Can you work these out from the drawing? Everything is in mm from the part's minimum corner. A direction names the side the tool comes from. Coordinates: 2 decimals unless noted, no trailing zeros. Loops run counter-clockwise (first coordinate to the right, second up) from the corner with the lowest first, then second, coordinate; pieces in that order, holes last.
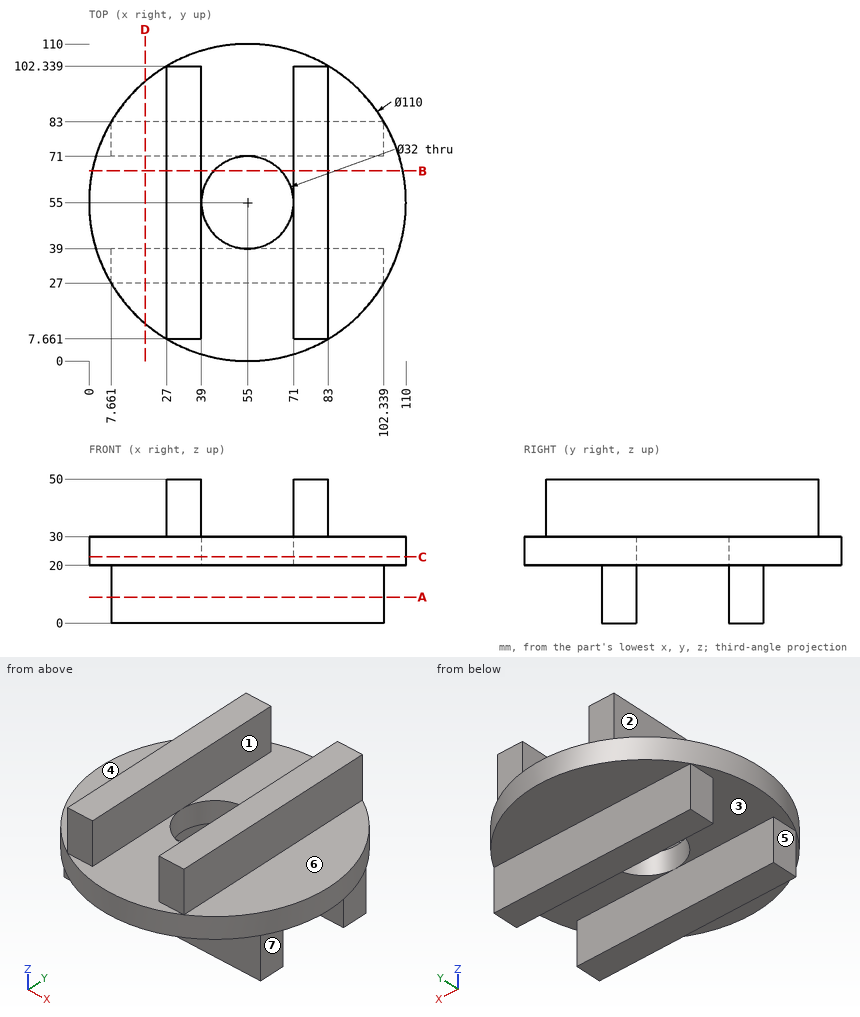
Item 1: Suppose I cut it at A-A, the plane z = 9. Please give me the cut outline in (x, y), plus the area to 3 significant figures.
Results are:
outline: (7.66, 27) - (102.34, 27) - (102.34, 39) - (7.66, 39) - close; (7.66, 71) - (102.34, 71) - (102.34, 83) - (7.66, 83) - close
area: 2,270 mm2
Item 2: Suppose I cut it at D-D, the plane x = 19.5. Please give me the cut outline in (y, z), plus the area to 3 significant figures.
Results are:
outline: (12.99, 20) - (27, 20) - (27, 0) - (39, 0) - (39, 20) - (71, 20) - (71, 0) - (83, 0) - (83, 20) - (97.01, 20) - (97.01, 30) - (12.99, 30) - close
area: 1,320 mm2
Item 3: I need wall thicknesses on line 1 along X through (y, z) = (55, 27.5); line 2 along Y through (x, z) = (86.5, 16.5). Which ranges of each line are inside material? Lowest first, please.
Results are:
line 1: x = 0 to 39, 71 to 110
line 2: y = 27 to 39, 71 to 83
Item 4: I'm going to push flat-ended pins straight in: P1, Ø5, axis at x = 61.5, y = 86.5, coming from the -Z side; P2, Ø16, axis at x = 42, z = 7, coming from the -Y side; P3, Ø1, axis at x = 19, z = 24, coming from the -Y side. Where does each tip first touch, or does it pass through?
Results are:
P1: stops at z = 20
P2: stops at y = 27
P3: stops at y = 12.99
Item 5: On a 3-axis mill with a long thin cutter (end or side, diameter ignored), from which of +Z, -Z, +X, -X, +Y, -Y can I reach the whole of each face in a straight line? I mean the marked faces 4, 5, 6 and 7. Say none if no direction works.
Results are:
face 4: +Z, -X, +Y, -Y
face 5: -Z, -X, +Y, -Y
face 6: +Z, +X, +Y, -Y
face 7: -Z, +X, +Y, -Y
Item 6: Suppose I cut it at C-C, the plane z = 23. Please give me the cut outline in (x, y), plus the area to 3 significant figures.
Results are:
outline: circle Ø110 at (55, 55); hole circle Ø32 at (55, 55)
area: 8,700 mm2
Item 7: We'd pull the mould along X, two halves only. Please class the marked faces 1, 2 and 3: +X half, -X half, draft (parallel to the pull), parting line (faces both ways), or undercut.
Results are:
face 1: undercut
face 2: -X half
face 3: draft
Item 8: Suppose I cut it at B-B, the plane y = 66. Please give me the cut outline in (x, z).
Results are:
outline: (1.11, 20) - (43.38, 20) - (43.38, 30) - (39, 30) - (39, 50) - (27, 50) - (27, 30) - (1.11, 30) - close; (66.62, 20) - (108.89, 20) - (108.89, 30) - (83, 30) - (83, 50) - (71, 50) - (71, 30) - (66.62, 30) - close
